```python
from build123d import *

# Parameters (mm, degrees)
SKETCH2_W               = 54.61
SKETCH2_H               = 29.97
SKETCH2_W_2             = 7
SKETCH2_H_2             = 6.37
SKETCH2_W_3             = 4.5
SKETCH2_H_3             = 4.5
BOSS_EXTRUDE4_DEPTH     = 3
SKETCH3_W               = 7
SKETCH3_H               = 6.37
BOSS_EXTRUDE5_DEPTH     = 3
SKETCH4_W               = 4.5
SKETCH4_H               = 4.5
BOSS_EXTRUDE6_DEPTH     = 2
SKETCH6_W               = 3.19390973
SKETCH6_H               = 2.94
CUT_EXTRUDE1_DEPTH      = 6.66
CUT_EXTRUDE1_DEPTH_BACK = 25.31
CUT_EXTRUDE3_REACH      = 20.17
SKETCH10_R              = 1
CUT_EXTRUDE4_DEPTH      = 5
SKETCH12_R              = 1.25
CUT_EXTRUDE5_DEPTH      = 0.5


with BuildPart() as part:
    # Sketch2 → Boss-Extrude4 (new body)
    with BuildSketch(Plane(origin=(0, 0, 0), x_dir=(1, 0, 0), z_dir=(0, 1, 0))):
        with Locations((-10.436162564, 12.528789446)):
            Rectangle(SKETCH2_W, SKETCH2_H)
        with Locations((-41.241162564, 12.528789446)):
            Rectangle(SKETCH2_W_2, SKETCH2_H_2)
        with Locations((19.118837436, 5.453789446)):
            Rectangle(SKETCH2_W_3, SKETCH2_H_3)
        with Locations((19.118837436, 19.603789446)):
            Rectangle(SKETCH2_W_3, SKETCH2_H_3)
    extrude(amount=BOSS_EXTRUDE4_DEPTH)

    # Sketch3 → Boss-Extrude5 (add)
    with BuildSketch(Plane(origin=(0, 3, 0), x_dir=(1, 0, 0), z_dir=(0, 1, 0))):
        with Locations((-41.241162564, 12.528789446)):
            Rectangle(SKETCH3_W, SKETCH3_H)
    extrude(amount=BOSS_EXTRUDE5_DEPTH)

    # Sketch4 → Boss-Extrude6 (add)
    with BuildSketch(Plane(origin=(0, 3, 0), x_dir=(1, 0, 0), z_dir=(0, 1, 0))):
        with Locations((19.118837436, 19.603789446)):
            Rectangle(SKETCH4_W, SKETCH4_H)
        with Locations((19.118837436, 5.453789446)):
            Rectangle(SKETCH4_W, SKETCH4_H)
    extrude(amount=BOSS_EXTRUDE6_DEPTH)

    # Sketch6 → Cut-Extrude1 (cut, two sides)
    with BuildSketch(Plane.XY.offset(-3.203789446)) as cut_extrude1_sk:
        with Locations((18.465792301, 3.53)):
            Rectangle(SKETCH6_W, SKETCH6_H)
    extrude(amount=CUT_EXTRUDE1_DEPTH, mode=Mode.SUBTRACT)
    extrude(cut_extrude1_sk.sketch, amount=-CUT_EXTRUDE1_DEPTH_BACK, mode=Mode.SUBTRACT)

    # Sketch8 → Cut-Extrude3 (cut, up to next)
    with BuildSketch(Plane.XY.offset(-9.343789446), mode=Mode.PRIVATE) as cut_extrude3_sk1:
        Polygon((-37.741162564, 6), (-42.018009261, 6), (-42.018009261, 6.012510793), (-43.247603098, 6.012510793), (-43.247603098, 6.015261621), (-44.781895645, 6.015261621), (-44.781895645, 2.058576766), (-37.741162564, 2.058576766), align=None)
    cut_extrude3_tool1 = extrude(cut_extrude3_sk1.sketch, amount=-CUT_EXTRUDE3_REACH, mode=Mode.PRIVATE) & part.part
    add(cut_extrude3_tool1.solids().sort_by_distance((-41.264608, 4.03205, -9.343789))[0], mode=Mode.SUBTRACT)

    # Sketch10 → Cut-Extrude4 (cut)
    with BuildSketch(Plane.XZ):
        with Locations((-41.551162564, -12.528789446)):
            Circle(SKETCH10_R)
    extrude(amount=-CUT_EXTRUDE4_DEPTH, mode=Mode.SUBTRACT)

    # Sketch12 → Cut-Extrude5 (cut)
    with BuildSketch(Plane.XZ):
        with Locations((-41.551162564, -12.528789446)):
            Circle(SKETCH12_R)
    extrude(amount=-CUT_EXTRUDE5_DEPTH, mode=Mode.SUBTRACT)


solid = part.part
```
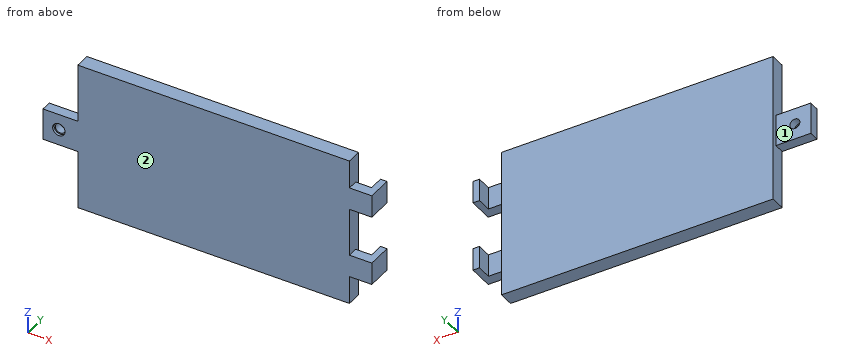
The listing builds one solid part. Answer for the finished solid, in the listing's coordinates (mm). Face numbers are marked on the shaded views. A direction names the side the tool comes from. Coordinates: 2 decimals unless noted, no trailing zeros. Write each loop counter-clockwise with the first axis right and the second up, starting at its lowest first coordinate (ties: lowest second). Pieces come first, ordered by that corner, then holes.
Q1. Find the intervals of material crossed by line 1 along X through (y, z) = (1, -12.5); line 2 along X through (y, z) = (2.75, -18.75); line 3 along Y through (x, z) = (-28.5, -26.5), in increasing order.
Returned:
line 1: x = -44.74 to -42.55, -40.55 to 16.87
line 2: x = -37.74 to 16.87, 20.06 to 21.37
line 3: y = 0 to 3
Q2. Section B-B, the plane z = -21.25 is taken. Write down the section's boundary in (x, y), then the cut area to 3 significant figures.
Returned:
outline: (-37.74, 0) - (21.37, 0) - (21.37, 5) - (20.06, 5) - (20.06, 2.06) - (16.87, 2.06) - (16.87, 3) - (-37.74, 3) - close
area: 177 mm2
Q3. Given P1, Ø1, axis at x = -42.5, y = 1, coming from the -Z side; P2, Ø6, axis at x = -6.5, z = -17, coming from the +Y side; P3, Ø1.6, axis at x = -41, y = 0.5, coming from the +Z side, each flat-ended and moving along its own axis, determine where each tip first touches the part or whether it passes through.
Returned:
P1: stops at z = -15.71
P2: stops at y = 3
P3: stops at z = -9.34
Q4. Which of the six approach directions +Z, -Z, +X, -X, +Y, -Y give full straight-line access (tool end or side, diameter ignored) to the marked faces 1 and 2?
Returned:
face 1: +Z, -Z, -X, +Y
face 2: +Z, -Z, +X, -X, -Y
Q5. Section A-A, the plane y = 3.6 is taken. Write down the section's boundary in (x, z), then the cut area to 3 significant figures.
Returned:
outline: (20.06, -21.85) - (21.37, -21.85) - (21.37, -17.35) - (20.06, -17.35) - close; (20.06, -7.7) - (21.37, -7.7) - (21.37, -3.2) - (20.06, -3.2) - close
area: 11.8 mm2
Q6. Section D-D, the plane z = -25.25 is taken. Write down the section's boundary in (x, y), then the cut area to 3 significant figures.
Returned:
outline: (-37.74, 0) - (16.87, 0) - (16.87, 3) - (-37.74, 3) - close
area: 164 mm2
Q7. Section C-C, the plane x = -19 is taken. Write down the section's boundary in (y, z).
Returned:
outline: (0, -27.51) - (3, -27.51) - (3, 2.46) - (0, 2.46) - close
